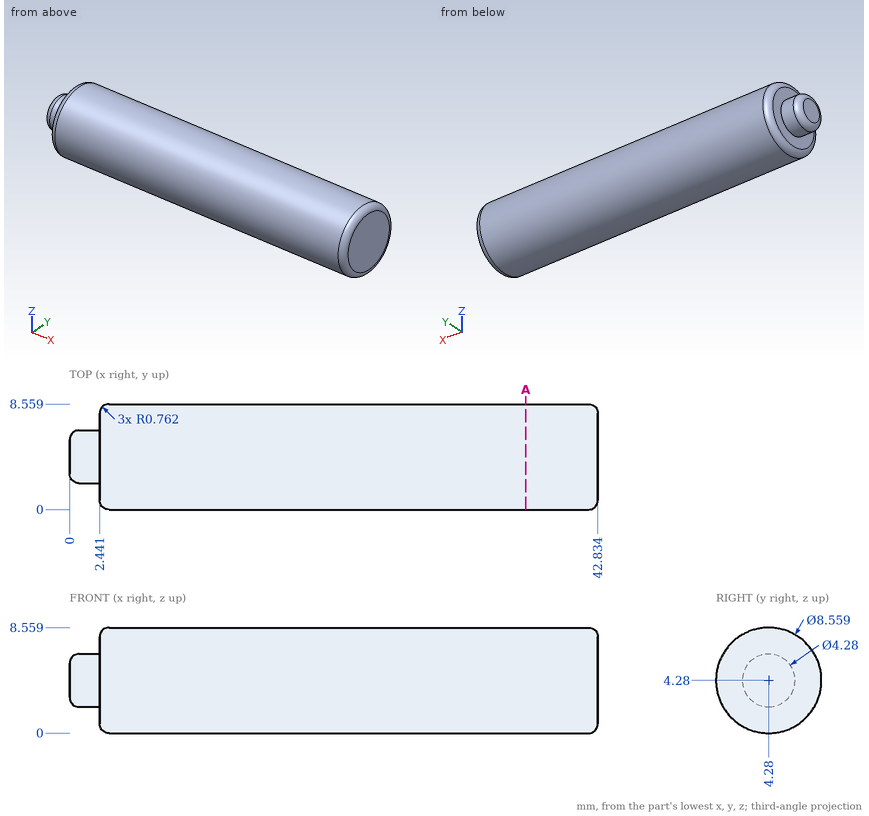
Design review of the part shown in the three views and the two pictorial views. Dimensions are in mm from the part's minimum x, y and z. Round coordinates to 2 decimals unless told otherwise and drop trailing zeros. Order: outer loops, then holes, each group sorted by start corner. A loop starts at its lowest first (then second) coordinate and runs counter-clockwise, first axis right, second up.
Q1. Insertion check: P1, Ø2, axis at x = 27.5, y = 6, coming from the +Z side. The pin has a flat end and moves straight along its axis. Give the tip position at first contact, or say it passes through.
Findings below:
P1: stops at z = 8.5
Q2. Wall thickness on line 1 (X direction, y = 2, z = 6.75); line 2 (X direction, y = 6.25, z = 7.5) (1 decimal); line 3 (Z direction, x = 37, y = 3) (1 decimal): over which ranges is each line inside the solid? List them lowest first.
Findings below:
line 1: x = 2.44 to 42.83
line 2: x = 2.5 to 42.8
line 3: z = 0.2 to 8.4
Q3. We need section A-A, the plane x = 37. Give the boundary of the cut face in (y, z).
Findings below:
outline: circle Ø8.56 at (4.28, 4.28)
